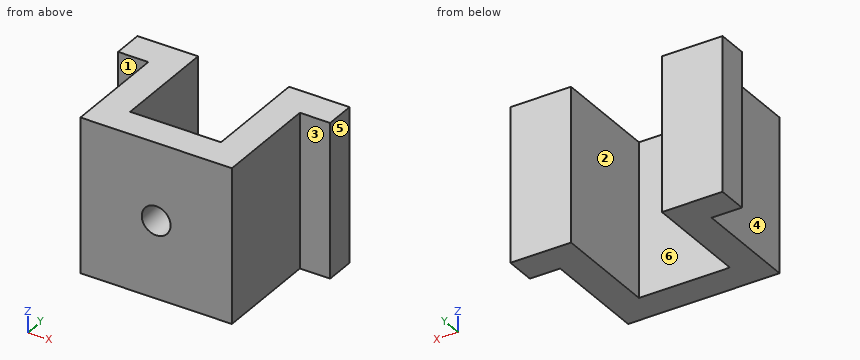
from build123d import *

# Parameters (mm, degrees)
EXTRUIR_L_MINA1_DEPTH = 25.4
CROQUIS2_R            = 4.7625
CORTAR_EXTRUIR1_DEPTH = 74.960530014


with BuildPart() as part:
    # Croquis1 → Extruir-Lámina1 (new, symmetric)
    with BuildSketch(Plane.XY):
        Polygon((-10, 35), (0, 35), (0, 0), (50, 0), (50, 35), (60, 35), (60, 45), (40, 45), (40, 10), (10, 10), (10, 45), (-10, 45), align=None)
    extrude(amount=EXTRUIR_L_MINA1_DEPTH, both=True)

    # Croquis2 → Cortar-Extruir1 (cut, through all)
    with BuildSketch(Plane(origin=(0, 10, 0), x_dir=(1, 0, 0), z_dir=(0, 1, 0))):
        with Locations(Location((25, 0, 0), (0, 0, 270))):
            Circle(CROQUIS2_R)
    extrude(amount=-CORTAR_EXTRUIR1_DEPTH, mode=Mode.SUBTRACT)


solid = part.part
Check sheet for the modelled part. Datum: model origin and axes. Units: mm. Face numbers are marked on the shaded views. A direction names the side the tool comes from. Give positions to 0.01 mm unless a question says otherwise; leave off trailing zeros. Loops run counter-clockwise (first coordinate to the right, second up) from the corner with the lowest first, then second, coordinate; pieces in that order, holes last. Notation, with made-up numbers: M 36.5,51 L 67.5,51 A20 cw 67.5,62 Z; hole C -8.75,40 d9. An arc over 180 degrees is marked long. Return JSON: item names as keys, results as strings. Group by question number.
1. Mould release check, pull along X, two halves, no side actions. Record for the marked faces 4, 5 and 6: released by +X, released by -X, zero draft, split by the parting line, or undercut.
2. Go/stop test with flat-tipped pins: pin 1 (17.5 mm diameter, centred on y = 16, z = -1.5, fed in from +X); pin 2 (10.5 mm diameter, centred on y = 14.5, z = 3, fed in from -X); pin 3 (3 mm diameter, centred on x = 56.5, z = -11.5, fed in from -Y). Record where each tip stops, or that it passes through.
3. Tool access check on the marked faces 1, 2 and 3. Record the directions out of +Z, -Z, +X, -X, +Y, -Y that give a thin tool (end or side, any length) a straight path to the whole face; none if there is none.
4. Thickness scan on L1, parallel to X at y = 2, z = 0; L2, parallel to X at y = 19, z = 0.5; L3, parallel to Y at x = 23, z = 11. Record the ranges inside material, lowest first.
5. Cross-section at B-B on x = 25. Record the boundary of the cut face in (y, z).
6. Cross-section at D-D on z = -9.5. Record the boundary of the cut face in (x, y).
7. Cross-section at C-C on z = 0. Record the boundary of the cut face in (x, y), plus the area to 3 significant figures.
8. Cross-section at A-A on y = 38. Record the boundary of the cut face in (x, z).
Return value:
{
 "1": {"face 4": "released by -X", "face 5": "released by +X", "face 6": "undercut"},
 "2": {"pin 1": "x = 50", "pin 2": "x = 0", "pin 3": "y = 35"},
 "3": {"face 1": "+Z, -Z, -X, -Y", "face 2": "+Z, -Z, +Y", "face 3": "+Z, -Z, +X, -Y"},
 "4": {"L1": "0 to 20.24, 29.76 to 50", "L2": "0 to 10, 40 to 50", "L3": "0 to 10"},
 "5": {"outline": "M 0,-25.4 L 10,-25.4 L 10,-4.76 L 0,-4.76 Z; M 0,4.76 L 10,4.76 L 10,25.4 L 0,25.4 Z"},
 "6": {"outline": "M -10,35 L 0,35 L 0,0 L 50,0 L 50,35 L 60,35 L 60,45 L 40,45 L 40,10 L 10,10 L 10,45 L -10,45 Z"},
 "7": {"outline": "M -10,35 L 0,35 L 0,0 L 20.24,0 L 20.24,10 L 10,10 L 10,45 L -10,45 Z; M 29.76,0 L 50,0 L 50,35 L 60,35 L 60,45 L 40,45 L 40,10 L 29.76,10 Z", "area": "1,300 mm^2"},
 "8": {"outline": "M -10,-25.4 L 10,-25.4 L 10,25.4 L -10,25.4 Z; M 40,-25.4 L 60,-25.4 L 60,25.4 L 40,25.4 Z"}
}
